CAD build for the part. Positions are in the model's coordinates, mm. Coordinates: 2 decimals unless noted, no trailing zeros. Order: outer loops, then holes, each group sorted by start corner. A loop starts at its lowest first (then second) coordinate and runs counter-clockwise, first axis right, second up. Notation, with made-up numbers: (86, -31) - (91, -31) arc R26 cw to (91, -14) - close; hole circle Ø7 at (27, 38). An arc over 180 degrees is marked (long way). Return JSON: item names as keys, results as strings.
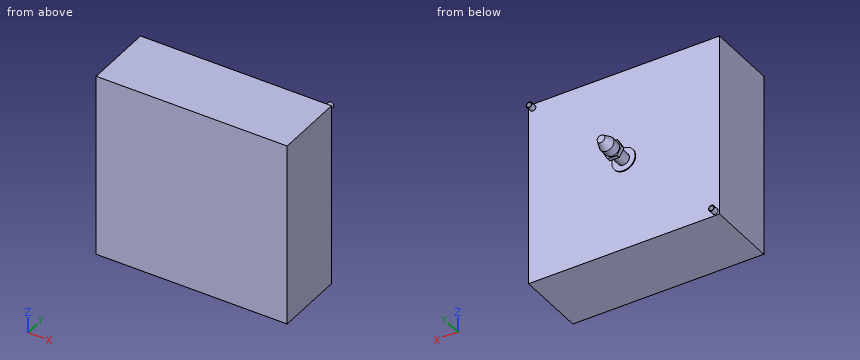
from build123d import *

# Parameters (mm, degrees)
SKETCH1_W      = 410
SKETCH1_H      = 150
EXTRUDE1_DEPTH = 197.5
SKETCH2_R      = 6.35
EXTRUDE2_DEPTH = 12.7
SHELL1_T       = -1
SKETCH3_R      = 25
EXTRUDE3_DEPTH = 2
SKETCH4_R      = 12.7
EXTRUDE4_DEPTH = 30
EXTRUDE5_DEPTH = 8


with BuildPart() as part:
    # Sketch1 → Extrude1 (new, symmetric)
    with BuildSketch(Plane.XY):
        with Locations((0, 75)):
            Rectangle(SKETCH1_W, SKETCH1_H)
    extrude(amount=EXTRUDE1_DEPTH, both=True)

    # Sketch2 → Extrude2 (add)
    with BuildSketch(Plane(origin=(0, 150, 0), x_dir=(1, 0, 0), z_dir=(0, 1, 0))):
        with Locations(Location((-195.680339288, 188.521302485, 0), (0, 0, 90))):
            Circle(SKETCH2_R)
        with Locations(Location((195.680339288, -188.521302485, 0), (0, 0, 90))):
            Circle(SKETCH2_R)
    extrude(amount=EXTRUDE2_DEPTH)

    # Shell1
    shell1_openings = [part.faces().sort_by_distance(p)[0] for p in [
        (-195.680339288, 162.7, -188.521302485),
        (195.680339288, 162.7, 188.521302485),
    ]]
    offset(amount=SHELL1_T, openings=shell1_openings, kind=Kind.INTERSECTION)

    # Sketch3 → Extrude3 (add)
    with BuildSketch(Plane(origin=(0, 150, 0), x_dir=(1, 0, 0), z_dir=(0, 1, 0))):
        with Locations(Location((0, 0, 0), (0, 0, 90))):
            Circle(SKETCH3_R)
    extrude(amount=EXTRUDE3_DEPTH)

    # Sketch4 → Extrude4 (add)
    with BuildSketch(Plane(origin=(0, 152, 0), x_dir=(1, 0, 0), z_dir=(0, 1, 0))):
        with Locations(Location((0, 0, 0), (0, 0, 270))):
            Circle(SKETCH4_R)
    extrude(amount=EXTRUDE4_DEPTH)

    # Sketch5 → Extrude5 (add)
    with BuildSketch(Plane(origin=(0, 182, 0), x_dir=(1, 0, 0), z_dir=(0, 1, 0))):
        Polygon((10.396549201, 17.327582002), (-9.807851599, 17.667466721), (-20.204400801, 0.339884719), (-10.396549201, -17.327582002), (9.807851599, -17.667466721), (20.204400801, -0.339884719), align=None)
    extrude(amount=EXTRUDE5_DEPTH)

    # Sketch6 → Revolve1 (revolve)
    with BuildSketch(Plane.XY, mode=Mode.PRIVATE) as revolve1_sk:
        Polygon((0, 190), (15.875, 190), (15.875, 209.05), (8.255, 228.1), (0, 228.1), align=None)
    revolve(revolve1_sk.sketch.rotate(Axis((0, 0, 0), (0, 1, 0)), 90), axis=Axis((0, 0, 0), (0, 1, 0)))


solid = part.part
Item 1: Band-saw the part on A-A, the plane x = -155.5. List the corners of the cut face in (y, z).
Findings below:
{"outline": "(0, -197.5) - (150, -197.5) - (150, 197.5) - (0, 197.5) - close; hole (1, -196.5) - (149, -196.5) - (149, 196.5) - (1, 196.5) - close"}
Item 2: Band-saw the part on C-C, the plane x = 0. List the corners of the cut face in (y, z) (3 decimals).
Findings below:
{"outline": "(0, -197.5) - (150, -197.5) - (150, -25) - (152, -25) - (152, -12.7) - (182, -12.7) - (182, -17.502) - (190, -17.502) - (190, -15.875) - (209.05, -15.875) - (228.1, -8.255) - (228.1, 8.255) - (209.05, 15.875) - (190, 15.875) - (190, 17.502) - (182, 17.502) - (182, 12.7) - (152, 12.7) - (152, 25) - (150, 25) - (150, 197.5) - (0, 197.5) - close; hole (1, -196.5) - (149, -196.5) - (149, 196.5) - (1, 196.5) - close"}
Item 3: Drop flat-ended pins along their axis: P1, Ø25, axis at x = -7, z = -8, coming from the +Y side; P2, Ø4, axis at x = -130, z = 112.5, coming from the +Y side; P3, Ø4, axis at x = -196.5, z = -189.5, coming from the +Y side. Give the stop position or say it passes through.
Findings below:
{"P1": "stops at y = 228.1", "P2": "stops at y = 150", "P3": "stops at y = 1"}
Item 4: Wall check: L1, parallel to Y at x = 180.5, z = -118; L2, parallel to X at y = 77.5, z = -110; L3, parallel to Z at x = -173, y = 115. Give the ranges that are in metal, low to high. Write a range as [from, to].
Findings below:
{"L1": "y = [0, 1], [149, 150]", "L2": "x = [-205, -204], [204, 205]", "L3": "z = [-197.5, -196.5], [196.5, 197.5]"}
Item 5: Band-saw the part on B-B, the plane z = -32. List the corners of the cut face in (x, y), then the cut area to 3 significant figures.
Findings below:
{"outline": "(-205, 0) - (205, 0) - (205, 150) - (-205, 150) - close; hole (-204, 1) - (204, 1) - (204, 149) - (-204, 149) - close", "area": "1,120 mm²"}
